Design review of the part built by this model. Coordinates are the model's own, in mm. A direction names the side the tool comes from. Give positions to 0.01 mm unless a question says otherwise; leave off trailing zeros. Write each loop counter-clockwise with the first axis right and the second up, starting at its lowest first coordinate (ties: lowest second). Pieces come first, ordered by that corner, then holes. Notation, with made-up numbers: M -34,41 L 7,41 A14 cw 7,51 Z; hole C -9.75,30 d8. An arc over 180 degrees is marked long. Answer in a Markdown table with one row per item.
```python
from build123d import *

# Parameters (mm, degrees)
F0_R     = 25.5
F0_R_2   = 12.5
F1_DEPTH = 25
F2_T     = -2
F3_DEPTH = 25
F4_R     = 28.5
F4_R_2   = 25.5
F5_DEPTH = 2


with BuildPart() as f1:
    # F0 (on Top) → F1 (new body)
    with BuildSketch(Plane.XY):
        Circle(F0_R)
        Circle(F0_R_2, mode=Mode.SUBTRACT)
        Circle(F0_R_2)
    extrude(amount=F1_DEPTH)

    # F2
    f2_openings = [f1.faces().sort_by_distance(p)[0] for p in [
        (0, 0, 0),
    ]]
    offset(amount=F2_T, openings=f2_openings)

    # F0 (on Top) → F3 (cut, through all)
    with BuildSketch(Plane.XY):
        Circle(F0_R_2)
    extrude(amount=F3_DEPTH, mode=Mode.SUBTRACT)

    # F4 (on face) → F5 (join)
    with BuildSketch(Plane.XY.offset(25)):
        Circle(F4_R)
        Circle(F4_R_2, mode=Mode.SUBTRACT)
    extrude(amount=-F5_DEPTH)


solid = f1.part
```
1) Add section A-A (x = 0). Write out the cut boundary in (y, z).
Geometry says:
| item | result |
|---|---|
| outline | M -28.5,23 L -25.5,23 L -25.5,0 L -23.5,0 L -23.5,23 L -12.5,23 L -12.5,25 L -28.5,25 Z; M 12.5,23 L 23.5,23 L 23.5,0 L 25.5,0 L 25.5,23 L 28.5,23 L 28.5,25 L 12.5,25 Z |
2) To check wall thickness, follow probe 1 along Y at (x, z) = (0, 23.6); probe 2 along Y at (x, z) = (-0.5, 6.25); probe 3 along Z at (x, y) = (2, -20). State the ranges of each line that lie inside material, in increasing order. Write a range as [from, to].
Geometry says:
| item | result |
|---|---|
| probe 1 | [-28.5, -12.5], [12.5, 28.5] |
| probe 2 | [-25.5, -23.49], [23.49, 25.5] |
| probe 3 | [23, 25] |
3) For faces 1 (the face through (11, -21, 0)), 2 (the face through (22.4, 7.1, 11.3)), list the 3-axis set-ups (+Z, -Z, +X, -X, +Y, -Y) from which the entire face can be reached by the end or side of a thin tool; tool diameter is ignored.
Geometry says:
| item | result |
|---|---|
| face 1 | -Z, +X, -X, +Y, -Y |
| face 2 | -Z |
4) The part is to be moulded in two halves that separate along X. For faces 3 (the face through (11.923, 3.755, 23.986)), 4 (the face through (12, -6, 25)), 5 (the face through (-5.5, -24.9, 11.3)), say which applies: released by +X, released by -X, zero draft, split by the parting line, or undercut.
Geometry says:
| item | result |
|---|---|
| face 3 | undercut |
| face 4 | zero draft |
| face 5 | split by the parting line |
5) Add section C-C (x = -22). Write out the cut boundary in (y, z).
Geometry says:
| item | result |
|---|---|
| outline | M -18.12,23 L -12.89,23 L -12.89,0 L -8.26,0 L -8.26,23 L 8.26,23 L 8.26,0 L 12.89,0 L 12.89,23 L 18.12,23 L 18.12,25 L -18.12,25 Z |
6) Add section D-D (z = 19.75). Write out the cut boundary in (x, y).
Geometry says:
| item | result |
|---|---|
| outline | C 0,0 d51; hole C 0,0 d47 |
7) Insertion check: P1, Ø4, axis at y = -21, z = 21.5, coming from the +X side; P2, Ø5, axis at x = 10.5, y = 15, coming from the -Z side; P3, Ø4, axis at x = -8, z = 9.5, coming from the +Y side. Each pin has a flat end and moves straight along its axis. Give the tip position at first contact, or say it passes through.
Geometry says:
| item | result |
|---|---|
| P1 | x = 20.62 |
| P2 | z = 23 |
| P3 | y = 24.78 |
